Check sheet for the modelled part. Datum: model origin and axes. Units: mm. A direction names the side the tool comes from. Round coordinates to 2 decimals unless told otherwise and drop trailing zeros. Write each loop counter-clockwise with the first axis right and the second up, starting at its lowest first coordinate (ties: lowest second). Pieces come first, ordered by that corner, then holes. Notation, with made-up numbers: M -8,10.5 L 32,10.5 A33 cw 32,43.5 Z; hole C -38,33.5 d2. An arc over 180 degrees is marked long. Answer in a Markdown table with one row per item.
```python
from build123d import *

# Parameters (mm, degrees)
SALIENTE_EXTRUIR1_DEPTH = 2
CROQUIS2_R              = 1.5
CORTAR_EXTRUIR1_DEPTH   = 7
CROQUIS3_R              = 4
CROQUIS3_R_2            = 3
SALIENTE_EXTRUIR2_DEPTH = 5


with BuildPart() as part:
    # Croquis1 → Saliente-Extruir1 (new, symmetric)
    with BuildSketch(Plane(origin=(0, 0, 0), x_dir=(1, 0, 0), z_dir=(0, 1, 0))):
        with BuildLine():
            Line((35, -28.516113802), (35, -4))
            Line((35, -4), (36.5, -4))
            Line((36.5, -4), (36.5, -7.5))
            ThreePointArc((36.5, -7.5), (37.5, -8.5), (38.5, -7.5))
            Line((38.5, -7.5), (38.5, 7.5))
            ThreePointArc((38.5, 7.5), (37.5, 8.5), (36.5, 7.5))
            Line((36.5, 7.5), (36.5, 4))
            Line((36.5, 4), (35, 4))
            Line((35, 4), (35, 28.516113802))
            ThreePointArc((35, 28.516113802), (35.879823326, 30.517678888), (37.949409202, 31.222779006))
            ThreePointArc((37.949409202, 31.222779006), (38.439227262, 31.49182987), (38.37918033, 32.047441664))
            ThreePointArc((38.37918033, 32.047441664), (-50, 0), (38.37918033, -32.047441664))
            ThreePointArc((38.37918033, -32.047441664), (38.439227262, -31.49182987), (37.949409202, -31.222779006))
            ThreePointArc((37.949409202, -31.222779006), (35.879823326, -30.517678888), (35, -28.516113802))
        make_face()
    extrude(amount=SALIENTE_EXTRUIR1_DEPTH, both=True)

    # Croquis2 → Cortar-Extruir1 (cut)
    with BuildSketch(Plane.XZ.offset(2)):
        with Locations(Location((17.5, 30.310889132, 0), (0, 0, 270))):
            Circle(CROQUIS2_R)
        with Locations(Location((-35, 0, 0), (0, 0, 270))):
            Circle(CROQUIS2_R)
        with Locations(Location((17.5, -30.310889132, 0), (0, 0, 270))):
            Circle(CROQUIS2_R)
    extrude(amount=-CORTAR_EXTRUIR1_DEPTH, mode=Mode.SUBTRACT)

    # Croquis3 → Saliente-Extruir2 (add)
    # profile 1 of 3: a face of its own
    with BuildSketch(Plane.XZ.offset(2)):
        with Locations(Location((-35, 0, 0), (0, 0, 90))):
            Circle(CROQUIS3_R)
        with Locations(Location((-35, 0, 0), (0, 0, 270))):
            Circle(CROQUIS3_R_2, mode=Mode.SUBTRACT)
    # profile 2 of 3: a face of its own
    with BuildSketch(Plane.XZ.offset(2)):
        with Locations(Location((17.5, 30.310889132, 0), (0, 0, 90))):
            Circle(CROQUIS3_R)
        with Locations(Location((17.5, 30.310889132, 0), (0, 0, 270))):
            Circle(CROQUIS3_R_2, mode=Mode.SUBTRACT)
    # profile 3 of 3: a face of its own
    with BuildSketch(Plane.XZ.offset(2)):
        with Locations(Location((17.5, -30.310889132, 0), (0, 0, 90))):
            Circle(CROQUIS3_R)
        with Locations(Location((17.5, -30.310889132, 0), (0, 0, 270))):
            Circle(CROQUIS3_R_2, mode=Mode.SUBTRACT)
    extrude(amount=SALIENTE_EXTRUIR2_DEPTH)


solid = part.part
```
1. Draft check along Z on faces 1 (the face through (36.5, 0, 6)), 2 (the face through (-38.966, -4.465, -0.521)), 3 (the face through (17, -7, -27)). Enter one of: +Z half, -Z half, draft (parallel to the pull), parting line (faces both ways), or undercut.
Found:
| item | result |
|---|---|
| face 1 | undercut |
| face 2 | parting line |
| face 3 | draft |
2. Section check D-D, the plane x = -35. Record the cut outline in (y, z), and give its area (3 significant figures).
Found:
| item | result |
|---|---|
| outline | M -7,-4 L -2,-4 L -2,-35.71 L 2,-35.71 L 2,-1.5 L -2,-1.5 L -2,-3 L -7,-3 Z; M -7,3 L -2,3 L -2,1.5 L 2,1.5 L 2,35.71 L -2,35.71 L -2,4 L -7,4 Z |
| area | 284 mm2 |
3. Scan lines: L1, parallel to X at y = -4.4, z = 0; L2, parallel to Y at x = -24, z = 6.5; L3, parallel to X at y = -0.25, z = 42.5. Record each from-to range of solid material in increasing order.
Found:
| item | result |
|---|---|
| L1 | x = -39 to -38, -32 to -31 |
| L2 | y = -2 to 2 |
| L3 | x = -26.34 to 26.34 |
4. Go/stop test with flat-tipped pins: pin 1 (3 mm diameter, centred on y = 0.5, z = 5, fed in from -X); pin 2 (4.5 mm diameter, centred on y = -0.5, z = 15, fed in from +X); pin 3 (2 mm diameter, centred on x = 11, z = 22, fed in from -Y); pin 4 (2.5 mm diameter, centred on x = 17.5, z = -30.31, fed in from -Y). Record where each tip stops, or that it passes through.
Found:
| item | result |
|---|---|
| pin 1 | stops at x = -49.88 |
| pin 2 | stops at x = 35 |
| pin 3 | stops at y = -2 |
| pin 4 | passes through |
5. Section check B-B, the plane z = 0. Record the cut outline in (x, y), and give its area (3 significant figures).
Found:
| item | result |
|---|---|
| outline | M -50,-2 L -39,-2 L -39,-7 L -38,-7 L -38,-2 L -36.5,-2 L -36.5,2 L -50,2 Z; M -33.5,-2 L -32,-2 L -32,-7 L -31,-7 L -31,-2 L 38.5,-2 L 38.5,2 L -33.5,2 Z |
| area | 352 mm2 |
6. Section check A-A, the plane y = -3.5. Record the cut outline in (x, z), and give its area (3 significant figures).
Found:
| item | result |
|---|---|
| outline | C -35,0 d8; C 17.5,-30.31 d8; C 17.5,30.31 d8; hole C -35,0 d6; hole C 17.5,-30.31 d6; hole C 17.5,30.31 d6 |
| area | 66.0 mm2 |
7. Access from +Z, -Z, +X, -X, +Y, -Y to the whole of each face (thin tool, end or side, straight path). Record for faces 4 (the face through (-6, 2, -1)), 5 (the face through (17.63, -4.46, 33.31)), 6 (the face through (35, 0, -16)).
Found:
| item | result |
|---|---|
| face 4 | +Z, -Z, +X, -X, +Y |
| face 5 | -Y |
| face 6 | +Y, -Y |
8. Section check C-C, the plane x = 17.5. Record the cut outline in (y, z), and give its area (3 significant figures).
Found:
| item | result |
|---|---|
| outline | M -7,-34.31 L -2,-34.31 L -2,-46.84 L 2,-46.84 L 2,-31.81 L -2,-31.81 L -2,-33.31 L -7,-33.31 Z; M -7,-27.31 L -2,-27.31 L -2,-28.81 L 2,-28.81 L 2,28.81 L -2,28.81 L -2,27.31 L -7,27.31 L -7,26.31 L -2,26.31 L -2,-26.31 L -7,-26.31 Z; M -7,33.31 L -2,33.31 L -2,31.81 L 2,31.81 L 2,46.84 L -2,46.84 L -2,34.31 L -7,34.31 Z |
| area | 371 mm2 |
